Design review of the part built by this model. Coordinates are the model's own, in mm. Face numbers are marked on the shaded views. A direction names the side the tool comes from. Coordinates: 2 decimals unless noted, no trailing zeros. Loops run counter-clockwise (first coordinate to the right, second up) from the corner with the lowest first, then second, coordinate; pieces in that order, holes last. Notation, with made-up numbers: (-2.5, 62.5) -> (3.5, 62.5) arc R23 cw to (3.5, 70.5) -> close; hole circle Ø9 at (89, 27.25). An arc over 180 degrees is marked (long way). Use a Markdown table: item, result. Add a question column.
Q1. Take a section at A-A on x = -75. Write out the cut boundary in (y, z), plus the area to 3 significant figures.
Q2. Take a section at C-C on x = 46. Write out the cut boundary in (y, z), plus the area to 3 significant figures.
Q3. For the marked faces 1 and 2, list the 3-axis set-ups (+Z, -Z, +X, -X, +Y, -Y) from which the entire face can be reached by the end or side of a thin tool; tool diameter is ignored.
Q4. Clearance check with flat-ended pins moving along their axes: pin 1 Ø5 at (y, z) = (41, 15.5) entering from -X (3 decimals); pin 2 Ø10 at (x, y) = (-5, 71) entering from +Z; pin 3 Ø8 at (x, y) = (43.5, -35) entering from +Z. State where each tip first meets the part, or that it passes through.
Q5. Take a section at B-B on z = 13. Write out the cut boundary in (x, y) (3 decimals).
Q6. For probe 1 along Y at (x, z) = (0, 3.25); probe 2 along Y at (x, z) = (0, 12.5); probe 3 along Y at (x, z) = (9.5, 11.25), list the stretches that pass through material, from the lowest coordinate up.
from build123d import *

# Parameters (mm, degrees)
SKETCH_1_W                            = 110
SKETCH_1_H                            = 166
EXTRUDE_1_DEPTH                       = 10
SKETCH_2_W                            = 30
SKETCH_2_H                            = 20
EXTRUDE_2_DEPTH                       = 5.5
HOLE_WIZARD_2_D                       = 6.6
HOLE_WIZARD_2_CBORE_D                 = 11
HOLE_WIZARD_2_CBORE_DEPTH             = 8.8
FILLET_2_R                            = 15
FILLET_3_R                            = 5
SKETCH_9_W                            = 76
SKETCH_9_H                            = 114
CUT_EXTRUDE_1_DEPTH                   = 101.069975517
FILLET_4_R                            = 5
SKETCH_11_W                           = 32.752695491
SKETCH_11_H                           = 40
EXTRUDE_4_DEPTH                       = 10
HOLE_WIZARD_2_2_D                     = 6.4
HOLE_WIZARD_2_2_CBORE_D               = 11
HOLE_WIZARD_2_2_CBORE_DEPTH           = 6.8
HOLE_WIZARD_2_2_ON_FACE_2_D           = 6.4
HOLE_WIZARD_2_2_ON_FACE_2_CBORE_D     = 11
HOLE_WIZARD_2_2_ON_FACE_2_CBORE_DEPTH = 6.8
SKETCH_14_W                           = 11
SKETCH_14_H                           = 25
CUT_EXTRUDE_3_DEPTH                   = 6.8
FILLET_5_R                            = 5
SKETCH_16_W                           = 6.4
SKETCH_16_H                           = 25
CUT_EXTRUDE_5_DEPTH                   = 122.411801593
SKETCH_17_W                           = 10
SKETCH_17_H                           = 15
EXTRUDE_5_DEPTH                       = 5.971999808
EXTRUDE_START                         = -3.675
SKETCH_18_W                           = 15
SKETCH_18_H                           = 20
EXTRUDE_6_DEPTH                       = 3.675
FILLET_6_R                            = 5
FILLET_7_R                            = 2
MM_1_D                                = 4
MM_1_DEPTH                            = 5
MM_1_TIP                              = 1.201721238
CUT_EXTRUDE_6_DEPTH                   = 5
EXTRUDE_START_2                       = -10
EXTRUDE_7_DEPTH                       = 10
CHAMFER_1_SIZE                        = 10


with BuildPart() as part:
    # 草图1 → 凸台-拉伸1 (new body)
    with BuildSketch(Plane.XY):
        Rectangle(SKETCH_1_W, SKETCH_1_H)
    extrude(amount=EXTRUDE_1_DEPTH)

    # 草图2 → 凸台-拉伸2 (add)
    with BuildSketch(Plane.XY.offset(10)):
        with Locations((0, -73)):
            Rectangle(SKETCH_2_W, SKETCH_2_H)
        with Locations((0, 73)):
            Rectangle(SKETCH_2_W, SKETCH_2_H)
    extrude(amount=EXTRUDE_2_DEPTH)

    # Hole Wizard 2 (through all)
    with Locations(Plane(origin=(0, 0, 0), x_dir=(-1, 0, 0), z_dir=(0, 0, -1))):
        with Locations((0, -73.35), (0, 73.35)):
            CounterBoreHole(HOLE_WIZARD_2_D / 2, HOLE_WIZARD_2_CBORE_D / 2, HOLE_WIZARD_2_CBORE_DEPTH)

    # 圆角2
    fillet_2_edges = [part.edges().sort_by_distance(p)[0] for p in [
        (55, -83, 5),
        (-55, -83, 5),
        (-55, 83, 5),
        (55, 83, 5),
    ]]
    fillet(fillet_2_edges, radius=FILLET_2_R)

    # 圆角3
    fillet_3_edges = [part.edges().sort_by_distance(p)[0] for p in [
        (-15, -63, 12.75),
        (15, -63, 12.75),
        (-15, 63, 12.75),
        (15, 63, 12.75),
    ]]
    fillet(fillet_3_edges, radius=FILLET_3_R)

    # 草图9 → 切除-拉伸1 (cut, through all)
    with BuildSketch(Plane.XY.offset(10)):
        Rectangle(SKETCH_9_W, SKETCH_9_H)
    extrude(amount=-CUT_EXTRUDE_1_DEPTH, mode=Mode.SUBTRACT)

    # 圆角4
    fillet_4_edges = [part.edges().sort_by_distance(p)[0] for p in [
        (38, 57, 5),
        (38, -57, 5),
        (-38, -57, 5),
        (-38, 57, 5),
    ]]
    fillet(fillet_4_edges, radius=FILLET_4_R)

    # 草图11 → 凸台-拉伸4 (add)
    with BuildSketch(Plane.XY.offset(10)):
        with Locations((-71.376347745, 0)):
            Rectangle(SKETCH_11_W, SKETCH_11_H)
        with Locations((71.376347745, 0)):
            Rectangle(SKETCH_11_W, SKETCH_11_H)
    extrude(amount=-EXTRUDE_4_DEPTH)

    # Hole Wizard 2 2 (through all)
    with Locations(Plane(origin=(75, -12.5, 10), x_dir=(1, 0, 0), z_dir=(0, 0, 1))):
        with Locations((0, 0), (-150, 25), (-150, 0), (0, 25)):
            CounterBoreHole(HOLE_WIZARD_2_2_D / 2, HOLE_WIZARD_2_2_CBORE_D / 2, HOLE_WIZARD_2_2_CBORE_DEPTH)

    # Hole Wizard 2 2 on face 2 (through all)
    with Locations(Plane(origin=(-121.442232178, 88.770272999, 0), x_dir=(1, 0, 0), z_dir=(0, 0, 1))):
        with Locations((0, 0)):
            CounterBoreHole(HOLE_WIZARD_2_2_ON_FACE_2_D / 2, HOLE_WIZARD_2_2_ON_FACE_2_CBORE_D / 2, HOLE_WIZARD_2_2_ON_FACE_2_CBORE_DEPTH)

    # 草图14 → 切除-拉伸3 (cut)
    with BuildSketch(Plane.XY.offset(10)):
        with Locations((-75, 0)):
            Rectangle(SKETCH_14_W, SKETCH_14_H)
        with Locations((75, 0)):
            Rectangle(SKETCH_14_W, SKETCH_14_H)
    extrude(amount=-CUT_EXTRUDE_3_DEPTH, mode=Mode.SUBTRACT)

    # 圆角5
    fillet_5_edges = [part.edges().sort_by_distance(p)[0] for p in [
        (-87.752695491, 20, 5),
        (-87.752695491, -20, 5),
        (-55, -20, 5),
        (-55, 20, 5),
        (55, -20, 5),
        (87.752695491, -20, 5),
        (87.752695491, 20, 5),
        (55, 20, 5),
    ]]
    fillet(fillet_5_edges, radius=FILLET_5_R)

    # 草图16 → 切除-拉伸5 (cut, through all)
    with BuildSketch(Plane.XY.offset(3.2)):
        with Locations((-75, 0)):
            Rectangle(SKETCH_16_W, SKETCH_16_H)
        with Locations((75, 0)):
            Rectangle(SKETCH_16_W, SKETCH_16_H)
    extrude(amount=-CUT_EXTRUDE_5_DEPTH, mode=Mode.SUBTRACT)

    # 草图17 → 凸台-拉伸5 (add)
    with BuildSketch(Plane(origin=(0, -83, 0), x_dir=(1, 0, 0), z_dir=(0, 1, 0))):
        with Locations((-20, -17.5)):
            Rectangle(SKETCH_17_W, SKETCH_17_H)
        with Locations((20, -17.5)):
            Rectangle(SKETCH_17_W, SKETCH_17_H)
    extrude(amount=EXTRUDE_5_DEPTH)

    # 草图18 → 凸台-拉伸6 (add)
    with BuildSketch(Plane(origin=(55, 0, 0), x_dir=(0, 0, -1), z_dir=(1, 0, 0)).offset(EXTRUDE_START)):
        with Locations((-17.5, 40)):
            Rectangle(SKETCH_18_W, SKETCH_18_H)
        with Locations((-17.5, -40)):
            Rectangle(SKETCH_18_W, SKETCH_18_H)
    extrude(amount=EXTRUDE_6_DEPTH)

    # 圆角6
    fillet_6_edges = [part.edges().sort_by_distance(p)[0] for p in [
        (53.1625, 50, 25),
        (53.1625, 30, 25),
        (53.1625, -30, 25),
        (53.1625, -50, 25),
        (25, -80.014000096, 25),
        (15, -80.014000096, 25),
        (-15, -80.014000096, 25),
        (-25, -80.014000096, 25),
    ]]
    fillet(fillet_6_edges, radius=FILLET_6_R - 0.0001)  # a hair under: the kernel refuses the full size

    # 圆角7
    fillet_7_edges = [part.edges().sort_by_distance(p)[0] for p in [
        (-15, -77.028000192, 12.75),
        (15, -77.028000192, 12.75),
    ]]
    fillet(fillet_7_edges, radius=FILLET_7_R)

    # 大小mm 暗销孔1
    with Locations(Plane(origin=(65, 0, 0), x_dir=(-1, 0, 0), z_dir=(0, 0, -1))):
        with Locations((0, 0)):
            Hole(MM_1_D / 2, depth=MM_1_DEPTH)
            with Locations((0, 0, -(MM_1_DEPTH + MM_1_TIP / 2))):  # 118° drill point
                Cone(0, MM_1_D / 2, MM_1_TIP, mode=Mode.SUBTRACT)

    # 草图21 → 切除-拉伸6 (cut)
    with BuildSketch(Plane(origin=(0, 0, 0), x_dir=(-1, 0, 0), z_dir=(0, 0, -1))):
        with BuildLine():
            Line((65.5, -2), (64.5, -2))
            ThreePointArc((64.5, -2), (62.5, 0), (64.5, 2))
            Line((64.5, 2), (65.5, 2))
            ThreePointArc((65.5, 2), (67.5, 0), (65.5, -2))
        make_face()
    extrude(amount=-CUT_EXTRUDE_6_DEPTH, mode=Mode.SUBTRACT)

    # 草图23 → 凸台-拉伸7 (add)
    with BuildSketch(Plane.XY.offset(10).offset(EXTRUDE_START_2)):
        with BuildLine():
            Line((-40, 83), (-87.752695491, 83))
            Line((-87.752695491, 83), (-87.752695491, 15))
            ThreePointArc((-87.752695491, 15), (-86.288229397, 18.535533906), (-82.752695491, 20))
            Line((-82.752695491, 20), (-60, 20))
            ThreePointArc((-60, 20), (-56.464466094, 21.464466094), (-55, 25))
            Line((-55, 25), (-55, 68))
            ThreePointArc((-55, 68), (-50.606601718, 78.606601718), (-40, 83))
        make_face()
        with BuildLine():
            ThreePointArc((-82.752695491, -20), (-86.288229397, -18.535533906), (-87.752695491, -15))
            Line((-87.752695491, -15), (-87.752695491, -83))
            Line((-87.752695491, -83), (-40, -83))
            ThreePointArc((-40, -83), (-50.606601718, -78.606601718), (-55, -68))
            Line((-55, -68), (-55, -25))
            ThreePointArc((-55, -25), (-56.464466094, -21.464466094), (-60, -20))
            Line((-60, -20), (-82.752695491, -20))
        make_face()
        with BuildLine():
            Line((87.752695491, -83), (87.752695491, -15))
            ThreePointArc((87.752695491, -15), (86.288229397, -18.535533906), (82.752695491, -20))
            Line((82.752695491, -20), (60, -20))
            ThreePointArc((60, -20), (56.464466094, -21.464466094), (55, -25))
            Line((55, -25), (55, -30))
            Line((55, -30), (51.324999949, -30))
            Line((51.324999949, -30), (51.324999949, -50))
            Line((51.324999949, -50), (55, -50))
            Line((55, -50), (55, -68))
            ThreePointArc((55, -68), (50.606601718, -78.606601718), (40, -83))
            Line((40, -83), (87.752695491, -83))
        make_face()
        with BuildLine():
            Line((87.752695491, 83), (40, 83))
            ThreePointArc((40, 83), (50.606601718, 78.606601718), (55, 68))
            Line((55, 68), (55, 50))
            Line((55, 50), (51.324999949, 50))
            Line((51.324999949, 50), (51.324999949, 30))
            Line((51.324999949, 30), (55, 30))
            Line((55, 30), (55, 25))
            ThreePointArc((55, 25), (56.464466094, 21.464466094), (60, 20))
            Line((60, 20), (82.752695491, 20))
            ThreePointArc((82.752695491, 20), (86.288229397, 18.535533906), (87.752695491, 15))
            Line((87.752695491, 15), (87.752695491, 83))
        make_face()
    extrude(amount=EXTRUDE_7_DEPTH)

    # 倒角1
    chamfer_1_edges = [part.edges().sort_by_distance(p)[0] for p in [
        (-87.752695491, 83, 5),
        (-87.752695491, -83, 5),
        (87.752695491, -83, 5),
        (87.752695491, 83, 5),
    ]]
    chamfer(chamfer_1_edges, length=CHAMFER_1_SIZE)


solid = part.part
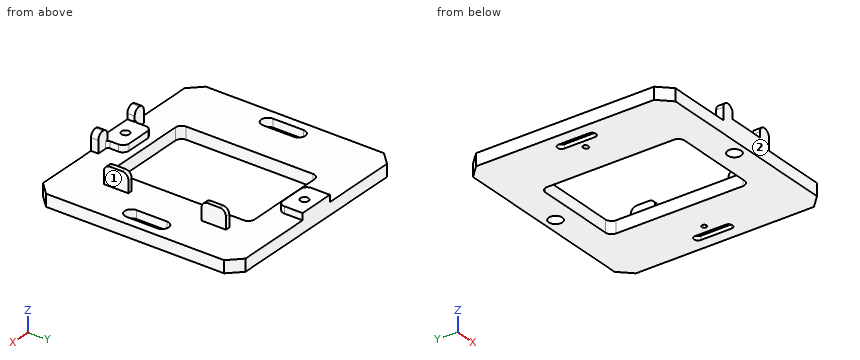
Answer list:
| question | item | result |
|---|---|---|
| 1 | outline | (-83, 0) -> (-15.7, 0) -> (-15.7, 3.2) -> (-18, 3.2) -> (-18, 10) -> (-83, 10) -> close; (15.7, 0) -> (83, 0) -> (83, 10) -> (18, 10) -> (18, 3.2) -> (15.7, 3.2) -> close |
| 1 | area | 1,310 mm² |
| 2 | outline | (-83, 0) -> (83, 0) -> (83, 10) -> (-83, 10) -> close |
| 2 | area | 1,660 mm² |
| 3 | face 1 | +Z, +X, +Y, -Y |
| 3 | face 2 | +Z, -Z, +X, -X, -Y |
| 4 | pin 1 | x = 51.325 |
| 4 | pin 2 | z = 15.5 |
| 4 | pin 3 | z = 10 |
| 5 | outline | (-25, -83) -> (25, -83) -> (25, -77.028) -> (17, -77.028) arc R2 cw to (15, -75.028) -> (15, -68) arc R5 ccw to (10, -63) -> (-10, -63) arc R5 ccw to (-15, -68) -> (-15, -75.028) arc R2 cw to (-17, -77.028) -> (-25, -77.028) -> close; (-15, 68) arc R5 ccw to (-10, 63) -> (10, 63) arc R5 ccw to (15, 68) -> (15, 83) -> (-15, 83) -> close; (51.325, -50) -> (55, -50) -> (55, -30) -> (51.325, -30) -> close; (51.325, 30) -> (55, 30) -> (55, 50) -> (51.325, 50) -> close; hole circle Ø6.6 at (0, -73.35); hole circle Ø6.6 at (0, 73.35) |
| 6 | probe 1 | -83 to -78.85, -67.85 to -57, 57 to 67.85, 78.85 to 83 |
| 6 | probe 2 | -83 to -76.65, -70.05 to -63, 63 to 70.05, 76.65 to 83 |
| 6 | probe 3 | -83 to -63, 63 to 83 |
